Autodesk Inventor part; units mm, degrees
ref_plane "YZ Plane" through (0, 0, 0) normal (1, 0, 0) x (0, 1, 0)
ref_plane "XZ Plane" through (0, 0, 0) normal (0, 1, 0) x (-1, 0, 0)
ref_plane "XY Plane" through (0, 0, 0) normal (0, 0, 1) x (1, 0, 0)
sketch "Sketch1" plane through (0, 0, 0) normal (0, 1, 0) x (-1, 0, 0)
  line L0 (20.32, 10.16) -> (-20.32, 10.16)
  line L1 (-20.32, 10.16) -> (-20.32, -10.16)
  line L2 (-20.32, -10.16) -> (20.32, -10.16)
  line L3 (20.32, -10.16) -> (20.32, 10.16)
  line L4 (22.225, 12.065) -> (-22.225, 12.065)
  line L5 (-22.225, 12.065) -> (-22.225, -12.065)
  line L6 (-22.225, -12.065) -> (22.225, -12.065)
  line L7 (22.225, -12.065) -> (22.225, 12.065)
  point P0 (0, 0)
  dimension "d0" = 40.64
  dimension "d1" = 20.32
  dimension "d2" = 40.64
  dimension "d3" = 44.45
  dimension "d4" = 24.13
  dimension "d5" = 44.45
extrude "Extrusion1" add sketch "Sketch1" along normal blind 56.515
sketch "Sketch2" plane through (-20.32, 0, -10.16) normal (1, 0, 0) x (0, 0, -1)
  line L0 (0, 0) -> (-20.32, 0)
  line L1 (0, 0) -> (0, 56.515)
  line L2 (-20.32, 56.515) -> (0, 56.515)
  line L3 (-20.32, 0) -> (-20.32, 56.515)
  point P0 (-10.16, 0)
extrude "Extrusion2" cut sketch "Sketch2" against normal blind 56.515
sketch "Sketch3" plane through (20.32, 0, 10.16) normal (-1, 0, 0) x (0, 0, 1)
  line L0 (0, 0) -> (-20.32, 0)
  line L1 (0, 0) -> (0, 56.515)
  line L2 (-20.32, 56.515) -> (0, 56.515)
  line L3 (-20.32, 0) -> (-20.32, 56.515)
  point P0 (-10.16, 0)
extrude "Extrusion3" cut sketch "Sketch3" against normal blind 56.515
sketch "Sketch4" plane through (22.225, 0, 10.16) normal (0, 0, -1) x (-1, 0, 0)
  line L0 (44.45, 56.515) -> (44.45, 0)
  line L1 (0, 56.515) -> (44.45, 56.515)
  line L2 (0, 0) -> (0, 56.515)
  line L3 (44.45, 54.61) -> (0, 54.61)
  point P0 (22.225, 0)
extrude "Extrusion4" add sketch "Sketch4" along normal blind 20.32
sketch "Sketch7" plane through (0, 56.515, 0) normal (0, 1, 0) x (1, 0, 0)
  circle A0 centre (18.415, 0) radius 1.5875
  circle A1 centre (5.715, 0) radius 1.5875
  circle A2 centre (-12.065, 0) radius 3.175
  point P0 (0, 0)
  dimension "d18" = 3.175
  dimension "d19" = 3.175
  dimension "d20" = 6.35
extrude "Extrusion7" cut sketch "Sketch7" against normal blind 15.24
sketch "Sketch10" plane through (0, 56.515, 0) normal (0, 1, 0) x (1, 0, 0)
  circle A0 centre (-12.065, 0) radius 3.175
  line L0 (-22.225, 12.065) -> (-22.225, -12.065)
  line L1 (-22.225, -12.065) -> (22.225, -12.065)
  line L2 (22.225, 12.065) -> (-22.225, 12.065)
  line L3 (1.905, 12.065) -> (1.905, -12.065)
  point P0 (0, 0)
extrude "Extrusion10" cut sketch "Sketch10" along normal blind 19.05
sketch "Sketch11" plane through (22.225, 0, 10.16) normal (1, 0, 0) x (0, 0, -1)
  line L0 (0, 0) -> (0, 54.61)
  line L1 (0, 54.61) -> (20.32, 54.61)
  line L2 (20.32, 54.61) -> (20.32, 0)
  line L3 (20.32, 0) -> (22.225, 0)
  line L4 (22.225, 0) -> (22.225, 56.515)
  line L5 (-1.905, 56.515) -> (22.225, 56.515)
  line L6 (-1.905, 0) -> (-1.905, 56.515)
  line L7 (-1.905, 0) -> (0, 0)
  line L8 (-1.905, 0) -> (-1.905, 56.515)
  line L9 (-1.905, 56.515) -> (-14.605, 56.515)
  line L10 (-14.605, 56.515) -> (-14.605, 0)
  line L11 (-14.605, 0) -> (-1.905, 0)
  line L12 (22.225, 0) -> (34.925, 0)
  line L13 (34.925, 0) -> (34.925, 56.515)
  line L14 (34.925, 56.515) -> (22.225, 56.515)
  line L15 (22.225, 0) -> (22.225, 56.515)
  line L16 (22.225, 0) -> (22.225, 56.515)
  line L17 (-14.605, 56.515) -> (-8.255, 56.515)
  circle A0 centre (-8.255, 10.5386) radius 2.286
  circle A1 centre (-8.255, 45.974) radius 2.286
  circle A2 centre (28.575, 45.974) radius 2.286
  circle A3 centre (28.575, 10.5386) radius 2.286
  point P0 (10.16, 0)
  dimension "d38" = 12.7
  dimension "d39" = 12.7
  dimension "d42" = 4.572
  dimension "d44" = 4.572
  dimension "d45" = 4.572
  dimension "d46" = 4.572
extrude "Extrusion11" add sketch "Sketch11" against normal blind 1.905 contours L11 L10 L9 L6 | L14 L13 L12 L4 | A0 | A1 | A2 | A3
extrude "Extrusion12" cut sketch "Sketch11" against normal blind 6.35 contours A0 | A1 | A2 | A3
properties part number "Autonomous - Ultrasonic Servo Mount V2"
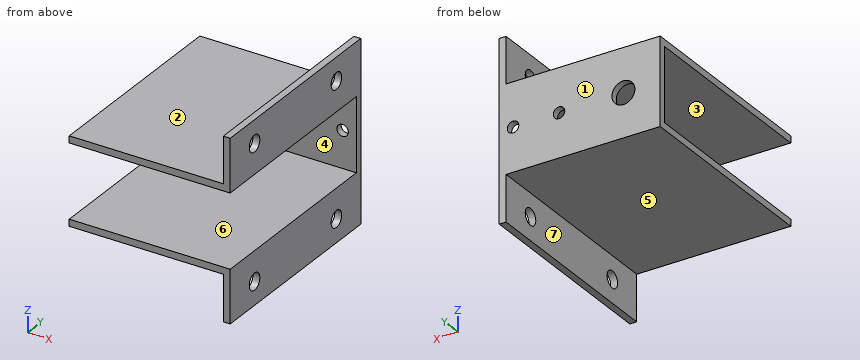
Here's how the part is built. I have some questions about the finished solid (model axes, mm). Face numbers are marked on the shaded views. A direction names the side the tool comes from. Round coordinates to 2 decimals unless told otherwise and drop trailing zeros. Loops run counter-clockwise (first coordinate to the right, second up) from the corner with the lowest first, then second, coordinate; pieces in that order, holes last. Notation, with made-up numbers: (-19.5, 19) - (8.5, 19) arc R23 cw to (8.5, 35) - close; hole circle Ø2 at (-9, -29). An arc over 180 degrees is marked (long way). One line per question, with ' | ' between items. Start each with the question number.
Q1. I want a section at D-D (z = -19.5). Write out the boundary of the cut face in (x, y) (1 decimal), then the cut area to 3 significant figures.
Q2. Please list where these lines run through material, in increasing order: line 1 (X direction, y = 55, z = 0) (1 decimal); line 2 (Z direction, x = 17.5, y = 45) (3 decimals); line 3 (Y direction, x = 9.5, z = 5) (3 decimals). Write a range as [from, to].
Q3. I want a section at B-B (y = 33). Write out the boundary of the cut face in (x, z) (3 decimals).
Q4. I want a section at C-C (x = 14). Write out the boundary of the cut face in (y, z) (3 decimals), then the cut area to 3 significant figures.
Q5. Will these pins go through, and if not, where does the flat tip stop? pin 1 (4 mm diameter, centred on x = 16, y = 38.5, fed in from -Z) (3 decimals); pin 2 (6 mm diameter, centred on x = -3.5, y = 32.5, fed in from +Z) (3 decimals); pin 3 (2 mm diameter, centred on x = -4, z = 4, fed in from -Y).
Q6. For the marked faces 1, 2 and 3, which set-ups out of +Z, -Z, +X, -X, +Y, -Y let a thin tool reach every point of the face, with its end or its side?
Q7. I want a section at A-A (z = 0). Write out the boundary of the cut face in (x, y) (1 decimal).
Q8. We'd pull the mould along Z, two halves only. Please class the marked faces 4, 5, 6 and 7: +Z half, -Z half, draft (parallel to the pull), parting line (faces both ways), or undercut.
Response values:
1) outline: (20.3, 0) - (22.2, 0) - (22.2, 8.5) - (20.3, 8.5) - close; (20.3, 12.6) - (22.2, 12.6) - (22.2, 44) - (20.3, 44) - close; (20.3, 48) - (22.2, 48) - (22.2, 56.5) - (20.3, 56.5) - close | area: 92.3 mm²
2) line 1: x = [-22.2, -15.2], [-8.9, 4.1], [7.3, 16.8], [20, 22.2] | line 2: z = [-12.065, -10.16], [10.16, 12.065] | line 3: y = [54.61, 56.515]
3) outline: (-22.225, -12.065) - (20.32, -12.065) - (20.32, -24.765) - (22.225, -24.765) - (22.225, -10.16) - (-22.225, -10.16) - close; (-22.225, 10.16) - (22.225, 10.16) - (22.225, 24.765) - (20.32, 24.765) - (20.32, 12.065) - (-22.225, 12.065) - close
4) outline: (0, -12.065) - (56.515, -12.065) - (56.515, 12.065) - (0, 12.065) - (0, 10.16) - (54.61, 10.16) - (54.61, -10.16) - (0, -10.16) - close | area: 254 mm²
5) pin 1: stops at z = -12.065 | pin 2: stops at z = 12.065 | pin 3: stops at y = 54.61
6) face 1: +Z, -Z, +X, -X, +Y | face 2: +Z, -X, +Y, -Y | face 3: +X, -X, -Y
7) outline: (-22.2, 54.6) - (-15.2, 54.6) - (-15.2, 56.5) - (-22.2, 56.5) - close; (-8.9, 54.6) - (4.1, 54.6) - (4.1, 56.5) - (-8.9, 56.5) - close; (7.3, 54.6) - (16.8, 54.6) - (16.8, 56.5) - (7.3, 56.5) - close; (20, 54.6) - (22.2, 54.6) - (22.2, 56.5) - (20, 56.5) - close
8) face 4: undercut | face 5: -Z half | face 6: undercut | face 7: draft
